Job drawing, mm, ordinate dimensions from the low corner. One solid piece. A direction names the side the tool comes from. Coordinates: 2 decimals unless noted, no trailing zeros. Order: outer loops, then holes, each group sorted by start corner. A loop starts at its lowest first (then second) coordinate and runs counter-clockwise, first axis right, second up. Notation, with made-up numbers: (45.25, 68.5) -> (73.25, 68.5) arc R14 ccw to (73.25, 90.5) -> close; hole circle Ø3 at (-36.75, 40). An arc over 180 degrees is marked (long way). Use CSV: the item, a comma, the result in double quotes. Start each with the question number.
(1) Tool access for the marked faces 1 and 2: list every direction of +Z, -Z, +X, -X, +Y, -Y with a clear straight run to the whole face (end or side of a thin tool).
(2) Probe L1, parallel to Y at x = 7.25, z = 1; L2, parallel to Z at x = 1.75, y = 2.85 (1 decimal); L3, parallel to X at y = 0.75, z = 6.75. List the from-to ranges inside material, lowest first.
(3) Cut at A-A on y = 2. Write the cut outline in (x, z).
(4) Pin check, flat tips, straight feed: pin 1 Ø1.5 at (y, z) = (1, 7) entering from +X; pin 2 Ø3 at (x, z) = (5, 2.5) entering from -Y. Stop position of each tip, or through.
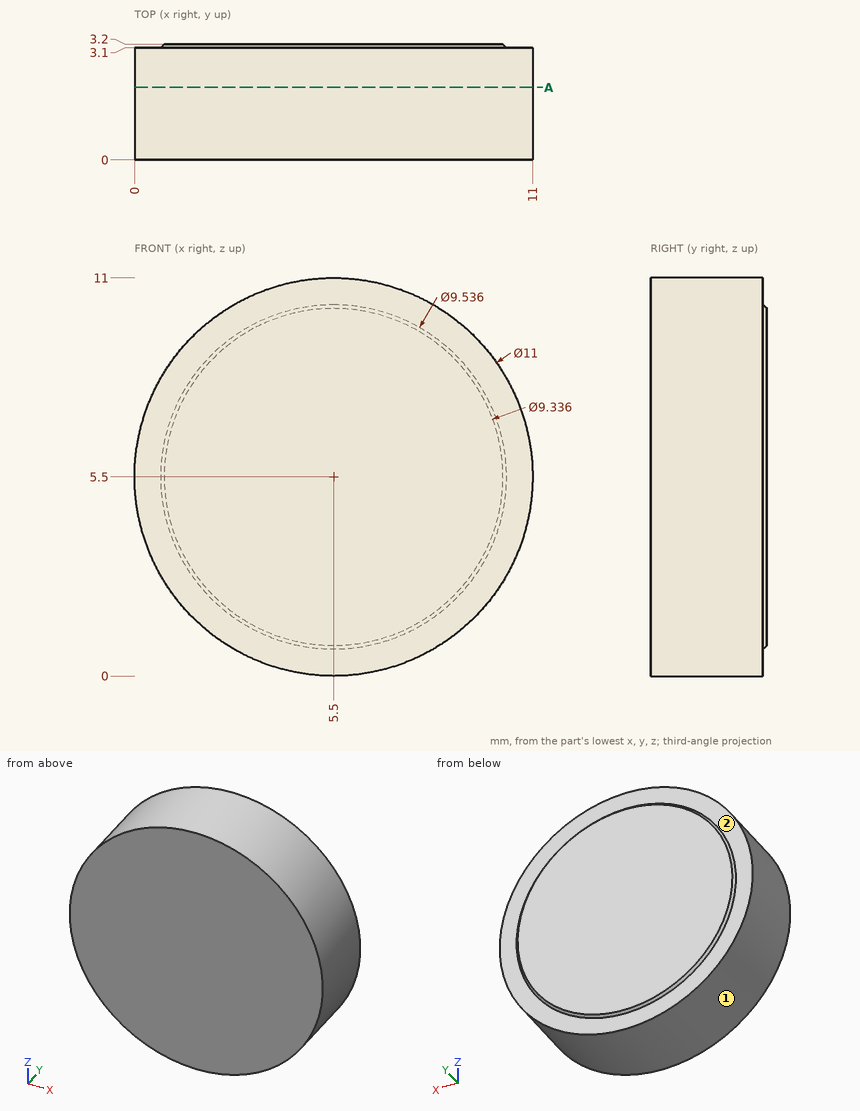
Outcome:
1,face 1,"+Y, -Y"
1,face 2,"+Y"
2,L1,"0 to 3.1"
2,L2,"1.5 to 9.5"
2,L3,"0.14 to 10.86"
3,outline,"circle Ø11 at (5.5, 5.5)"
4,pin 1,"x = 10.95"
4,pin 2,"y = 0"
